Geometry: final body of the model. Coordinates: model frame, mm. Face numbers are marked on the shaded views. A direction names the side the tool comes from. Give positions to 0.01 mm unless a question says otherwise; leave off trailing zeros. Write each loop counter-clockwise with the first axis right and the second up, starting at its lowest first coordinate (ties: lowest second). Pieces come first, ordered by that corner, then holes.
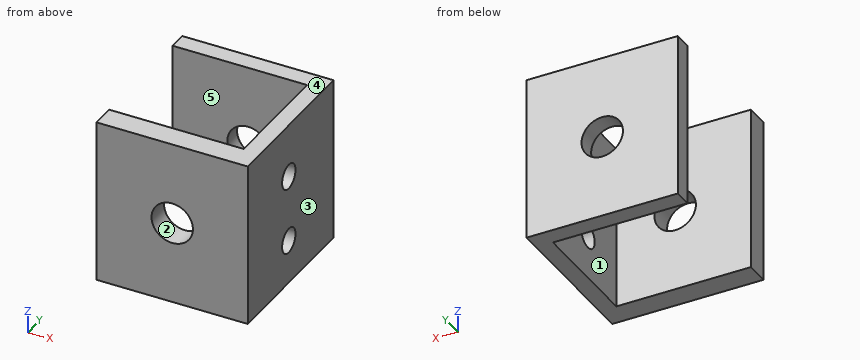
from build123d import *

# Parameters (mm, degrees)
ESQUISSE1_W             = 45.791168344
ESQUISSE1_H             = 48.162822482
BOSS_EXTRU_1_DEPTH      = 50
ESQUISSE6_W             = 40.720467392
ESQUISSE6_H             = 35.64976644
ENL_V_MAT_EXTRU_2_DEPTH = 84.165428922
ESQUISSE7_R             = 6.277140529
ENL_V_MAT_EXTRU_3_DEPTH = 84.165428922
ESQUISSE8_R             = 3.769419749
ENL_V_MAT_EXTRU_4_DEPTH = 81.484867733


with BuildPart() as part:
    # Esquisse1 → Boss.-Extru.1 (new body)
    with BuildSketch(Plane.XY):
        with Locations((22.895584172, 24.081411241)):
            Rectangle(ESQUISSE1_W, ESQUISSE1_H)
    extrude(amount=BOSS_EXTRU_1_DEPTH)

    # Esquisse6 → Enlèv. mat.-Extru.2 (cut, through all)
    with BuildSketch(Plane.XY.offset(50)):
        with Locations((20.360233696, 24.911961355)):
            Rectangle(ESQUISSE6_W, ESQUISSE6_H)
    extrude(amount=-ENL_V_MAT_EXTRU_2_DEPTH, mode=Mode.SUBTRACT)

    # Esquisse7 → Enlèv. mat.-Extru.3 (cut, through all)
    with BuildSketch(Plane(origin=(0, 48.162822482, 0), x_dir=(1, 0, 0), z_dir=(0, 1, 0))):
        with Locations(Location((22.895584172, -25, 0), (0, 0, 270))):
            Circle(ESQUISSE7_R)
    extrude(amount=-ENL_V_MAT_EXTRU_3_DEPTH, mode=Mode.SUBTRACT)

    # Esquisse8 → Enlèv. mat.-Extru.4 (cut, through all)
    with BuildSketch(Plane.ZY.offset(-40.720467392)):
        with Locations((13.372298401, 23.059195716)):
            Circle(ESQUISSE8_R)
        with Locations((33.688831964, 23.059195716)):
            Circle(ESQUISSE8_R)
    extrude(amount=-ENL_V_MAT_EXTRU_4_DEPTH, mode=Mode.SUBTRACT)


solid = part.part
Q1. Section D-D on y = 29. Output: boundary loops of the cut face in (x, z), plus the area to 3 significant figures.
Filled sheet:
outline: (40.72, 0) - (45.79, 0) - (45.79, 50) - (40.72, 50) - close
area: 254 mm2
Q2. Access query for the marked faces 4 and 5. Directions: +Z, -Z, +X, -X, +Y, -Y. A direction counts if a zero-diameter tool reaches every point of the face in a straight line with its end or side. Return the directions, or none.
Filled sheet:
face 4: +Z, +X, -X, +Y, -Y
face 5: +Z, -Z, -X
Q3. Section A-A on x = 15. Output: boundary loops of the cut face in (y, z), plus the area to 3 significant figures.
Filled sheet:
outline: (0, 0) - (7.09, 0) - (7.09, 50) - (0, 50) - close; (42.74, 0) - (48.16, 0) - (48.16, 50) - (42.74, 50) - close
area: 626 mm2
Q4. Pin query (flat end, axial travel): P1, Ø18, axis at y = 28, z = 29, coming from the -X side; P2, Ø12, axis at x = 11.5, z = 18, coming from the -Y side. Return the tip coordinate at first contact, or that it passes through.
Filled sheet:
P1: stops at x = 40.72
P2: stops at y = 0
Q5. Ray query, line 1 along Y through (x, z) = (34.5, 35); line 2 along X through (y, z) = (45, 25); line 3 along X through (y, z) = (38, 14.5). Return the intervals inside material, ascending.
Filled sheet:
line 1: y = 0 to 7.09, 42.74 to 48.16
line 2: x = 0 to 16.62, 29.17 to 45.79
line 3: x = 40.72 to 45.79
Q6. Section C-C on x = 21.5. Output: boundary loops of the cut face in (y, z), plus the area to 3 significant figures.
Filled sheet:
outline: (0, 0) - (7.09, 0) - (7.09, 18.88) - (0, 18.88) - close; (0, 31.12) - (7.09, 31.12) - (7.09, 50) - (0, 50) - close; (42.74, 0) - (48.16, 0) - (48.16, 18.88) - (42.74, 18.88) - close; (42.74, 31.12) - (48.16, 31.12) - (48.16, 50) - (42.74, 50) - close
area: 472 mm2
Q7. Section B-B on z = 25. Output: boundary loops of the cut face in (x, y).
Filled sheet:
outline: (0, 0) - (16.62, 0) - (16.62, 7.09) - (0, 7.09) - close; (0, 42.74) - (16.62, 42.74) - (16.62, 48.16) - (0, 48.16) - close; (29.17, 0) - (45.79, 0) - (45.79, 48.16) - (29.17, 48.16) - (29.17, 42.74) - (40.72, 42.74) - (40.72, 7.09) - (29.17, 7.09) - close
Q8. Pull-direction query (X, two-part tool) for the marked faces 1, 2 and 3; classes: released by +X, released by -X, zero draft, split by the parting line, or undercut.
Filled sheet:
face 1: released by -X
face 2: undercut
face 3: released by +X
